Source: CAD feature listing. Evaluate the final solid. Frame: model axes, mm. Round coordinates to 2 decimals unless told otherwise and drop trailing zeros. Write each loop counter-clockwise with the first axis right and the second up, starting at its lowest first coordinate (ties: lowest second). Pieces come first, ordered by that corner, then holes.
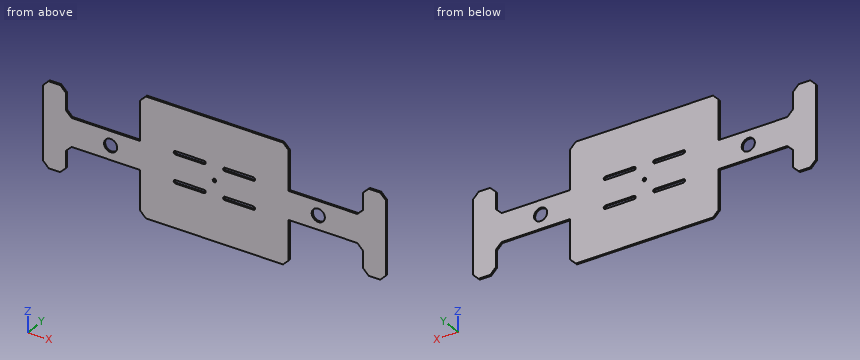
from build123d import *

# Parameters (mm, degrees)
SKETCH1_R           = 11.5
SKETCH1_R_2         = 3
BOSS_EXTRUDE1_DEPTH = 3


with BuildPart() as part:
    # Sketch1 → Boss-Extrude1 (new body)
    with BuildSketch(Plane(origin=(0, 0, 0), x_dir=(1, 0, 0), z_dir=(0, 1, 0))):
        Polygon((10, 150), (30, 150), (40, 140), (40, 110), (50, 100), (170, 100), (170, 170), (180, 180), (420, 180), (430, 170), (430, 100), (550, 100), (560, 110), (560, 140), (570, 150), (590, 150), (600, 140), (600, 10), (590, 0), (570, 0), (560, 10), (560, 40), (550, 50), (430, 50), (430, -20), (420, -30), (180, -30), (170, -20), (170, 50), (50, 50), (40, 40), (40, 10), (30, 0), (10, 0), (0, 10), (0, 140), align=None)
        with Locations(Location((118.3, 75, 0), (0, 0, 270))):
            Circle(SKETCH1_R, mode=Mode.SUBTRACT)
        with Locations(Location((481.7, 75, 0), (0, 0, 270))):
            Circle(SKETCH1_R, mode=Mode.SUBTRACT)
        with Locations(Location((300, 75, 0), (0, 0, 270))):
            Circle(SKETCH1_R_2, mode=Mode.SUBTRACT)
        with BuildLine():
            Line((231.666666667, 103), (281.666666667, 103))
            ThreePointArc((281.666666667, 103), (284.666666667, 100), (281.666666667, 97))
            Line((281.666666667, 97), (231.666666667, 97))
            ThreePointArc((231.666666667, 97), (228.666666667, 100), (231.666666667, 103))
        make_face(mode=Mode.SUBTRACT)
        with BuildLine():
            Line((318.333333333, 103), (368.333333333, 103))
            ThreePointArc((368.333333333, 103), (371.333333333, 100), (368.333333333, 97))
            Line((368.333333333, 97), (318.333333333, 97))
            ThreePointArc((318.333333333, 97), (315.333333333, 100), (318.333333333, 103))
        make_face(mode=Mode.SUBTRACT)
        with BuildLine():
            Line((231.666666667, 53), (281.666666667, 53))
            ThreePointArc((281.666666667, 53), (284.666666667, 50), (281.666666667, 47))
            Line((281.666666667, 47), (231.666666667, 47))
            ThreePointArc((231.666666667, 47), (228.666666667, 50), (231.666666667, 53))
        make_face(mode=Mode.SUBTRACT)
        with BuildLine():
            Line((318.333333333, 53), (368.333333333, 53))
            ThreePointArc((368.333333333, 53), (371.333333333, 50), (368.333333333, 47))
            Line((368.333333333, 47), (318.333333333, 47))
            ThreePointArc((318.333333333, 47), (315.333333333, 50), (318.333333333, 53))
        make_face(mode=Mode.SUBTRACT)
    extrude(amount=BOSS_EXTRUDE1_DEPTH)


solid = part.part
1) Section query B-B on x = 241.5. Return the cut outline in (y, z).
Taken from the geometry:
outline: (0, -180) - (3, -180) - (3, -103) - (0, -103) - close; (0, -97) - (3, -97) - (3, -53) - (0, -53) - close; (0, -47) - (3, -47) - (3, 30) - (0, 30) - close
2) Section query C-C on y = 0.75. State how many separate pieces and enclosed holes the cut face has, then the cut area to 3 significant figures.
Taken from the geometry:
separate pieces: 1
enclosed holes: 7
area: 77,000 mm2
3) Contact query for flat-ended pins moving along their axis: P1, Ø1.5, axis at x = 575.5, y = 2, coming from the +Z side; P2, Ø0.9, axis at x = 580.5, y = 2, coming from the -Z side. Output: stop coordinate, or through.
Taken from the geometry:
P1: stops at z = 0
P2: stops at z = -150
4) Material intervals for line 1 (X direction, y = 2.5, z = -26); line 2 (X direction, y = 1.75, z = -75); line 3 (Z direction, x = 243, y = 2), sorted ascending.
Taken from the geometry:
line 1: x = 0 to 40, 170 to 430, 560 to 600
line 2: x = 0 to 106.8, 129.8 to 297, 303 to 470.2, 493.2 to 600
line 3: z = -180 to -103, -97 to -53, -47 to 30
5) Section query A-A on x = 118.3. Return the cut outline in (y, z).
Taken from the geometry:
outline: (0, -100) - (3, -100) - (3, -86.5) - (0, -86.5) - close; (0, -63.5) - (3, -63.5) - (3, -50) - (0, -50) - close
